from build123d import *

# Parameters (mm, degrees)
F2_SIZE2   = 0.5358983849
F2_SIZE    = 2
F2_2_SIZE2 = 0.5358983849
F2_2_SIZE  = 2
F3_SIZE    = 0.5


with BuildPart() as f1:
    # F0 (on Front) → F1 (revolve)
    with BuildSketch(Plane.XZ):
        Polygon((0, 22.5), (0, 17.5), (50, 17.5), (50, 22), (40, 22), (40, 22.5), align=None)
    revolve(axis=Axis((25, 0, 0), (1, 0, 0)))

    # F2
    f2_edges = [f1.edges().sort_by_distance(p)[0] for p in [
        (0, 0, -17.5),
        (50, 0, -17.5),
    ]]
    f2_side = f1.faces().sort_by_distance((25, 0, -17.5))[0]
    chamfer(f2_edges, length=F2_SIZE, length2=F2_SIZE2, reference=f2_side)

    # F2#2
    f2_2_edges = [f1.edges().sort_by_distance(p)[0] for p in [
        (0, 0, -22.5),
    ]]
    f2_2_side = f1.faces().sort_by_distance((20, 0, -22.5))[0]
    chamfer(f2_2_edges, length=F2_2_SIZE, length2=F2_2_SIZE2, reference=f2_2_side)

    # F3
    f3_edges = [f1.edges().sort_by_distance(p)[0] for p in [
        (50, 0, -22),
    ]]
    chamfer(f3_edges, length=F3_SIZE)


solid = f1.part
Can you work these out from the model? Positions are in its coordinate system, mm. A direction names the side the tool comes from. Round coordinates to 2 decimals unless told otherwise and drop trailing zeros. Order: outer loops, then holes, each group sorted by start corner. A loop starts at its lowest first (then second) coordinate and runs counter-clockwise, first axis right, second up. Notation, with made-up numbers: (-23, 10) - (25, 10) arc R32 cw to (25, 37) - close; hole circle Ø1 at (-23, 61.5). An arc over 180 degrees is marked (long way). Answer in a Markdown table with one row per item.
(1) Which directions (+Z, -Z, +X, -X, +Y, -Y) give clear straight access to the entire face, cutting with the end or side of a thin tool? Please do faces 1 (the face through (50, -18, 5)), 2 (the face through (40, 9.9, -19.9)).
From the geometry:
| item | result |
|---|---|
| face 1 | +Z, -Z, +X, +Y, -Y |
| face 2 | +X |
(2) For P1, Ø6, axis at x = 9, z = -15.5, coming from the +Y side; P2, Ø10, axis at y = 9.5, z = 14, coming from the +X side; P3, Ø1, axis at x = 24.5, z = -11.5, coming from the -Y side; P4, Ø3, axis at x = 17.5, y = -17, coming from the +Z side, each with a flat end and sliding along its axis, tell me the tip position at first contact or that it passes through.
From the geometry:
| item | result |
|---|---|
| P1 | stops at y = 18.71 |
| P2 | stops at x = 50 |
| P3 | stops at y = -19.63 |
| P4 | stops at z = 16.31 |
(3) Please list where these lines run through material, in increasing order: L1, parallel to Z at x = 35.5, y = 0; L2, parallel to Y at x = 34, z = 9. Write a range as from..to.
From the geometry:
| item | result |
|---|---|
| L1 | z = -22.5..-17.5, 17.5..22.5 |
| L2 | y = -20.62..-15.01, 15.01..20.62 |
(4) Suppose I cut it at C-C, the plane x = 6. Please give me the cut outline in (y, z).
From the geometry:
| item | result |
|---|---|
| outline | circle Ø45 at (0, 0); hole circle Ø35 at (0, 0) |
(5) If we mould it in two halves opening along Y, with no side actions, what happens to faces 3 (the face through (25.322, 10.648, -13.887)), 4 (the face through (0, -18, -3)), 5 (the face through (44.684, 21.477, -4.769))? For each: released by +Y, released by -Y, zero draft, split by the parting line, or undercut.
From the geometry:
| item | result |
|---|---|
| face 3 | undercut |
| face 4 | zero draft |
| face 5 | split by the parting line |
(6) Suppose I cut it at A-A, the plane z = 0. Please give me the cut outline in (x, y).
From the geometry:
| item | result |
|---|---|
| outline | (0, -21.96) - (2, -22.5) - (40, -22.5) - (40, -22) - (49.5, -22) - (50, -21.5) - (50, -18.04) - (48, -17.5) - (2, -17.5) - (0, -18.04) - close; (0, 18.04) - (2, 17.5) - (48, 17.5) - (50, 18.04) - (50, 21.5) - (49.5, 22) - (40, 22) - (40, 22.5) - (2, 22.5) - (0, 21.96) - close |
